Part model, mm, in its own coordinate system. Face numbers are marked on the shaded views. A direction names the side the tool comes from. Round coordinates to 2 decimals unless told otherwise and drop trailing zeros. Loops run counter-clockwise (first coordinate to the right, second up) from the corner with the lowest first, then second, coordinate; pieces in that order, holes last. Notation, with made-up numbers: (-34, 4.5) - (3, 4.5) arc R12 ccw to (3, 8.5) - close; hole circle Ø9 at (19.5, 64). An arc over 180 degrees is marked (long way). Put each result on its own line as item: value.
from build123d import *

# Parameters (mm, degrees)
CUT_EXTRUDE1_DEPTH = 15


with BuildPart() as part:
    # Sketch1 → Revolve1 (revolve)
    with BuildSketch(Plane.XY):
        Polygon((-3, 0), (-3, 7), (-9, 7), (0, 40), (0, 0), align=None)
    revolve(axis=Axis((0, 40, 0), (0, -1, 0)))

    # Sketch2 → Cut-Extrude1 (cut)
    with BuildSketch(Plane.XZ.offset(-7)):
        with BuildLine():
            Line((-2.079651877, 8.756428956), (0, 5.274248167))
            Line((0, 5.274248167), (2.079651877, 8.756428956))
            ThreePointArc((2.079651877, 8.756428956), (0, 9.330174076), (-2.079651877, 8.756428956))
        make_face()
        with BuildLine():
            Line((8.756428956, 2.079651877), (5.274248167, 0))
            Line((5.274248167, 0), (8.756428956, -2.079651877))
            ThreePointArc((8.756428956, -2.079651877), (9.330174076, 0), (8.756428956, 2.079651877))
        make_face()
        with BuildLine():
            Line((2.079651877, -8.756428956), (0, -5.274248167))
            Line((0, -5.274248167), (-2.079651877, -8.756428956))
            ThreePointArc((-2.079651877, -8.756428956), (0, -9.330174076), (2.079651877, -8.756428956))
        make_face()
        with BuildLine():
            Line((-8.756428956, -2.079651877), (-5.274248167, 0))
            Line((-5.274248167, 0), (-8.756428956, 2.079651877))
            ThreePointArc((-8.756428956, 2.079651877), (-9.330174076, 0), (-8.756428956, -2.079651877))
        make_face()
    extrude(amount=-CUT_EXTRUDE1_DEPTH, mode=Mode.SUBTRACT)


solid = part.part
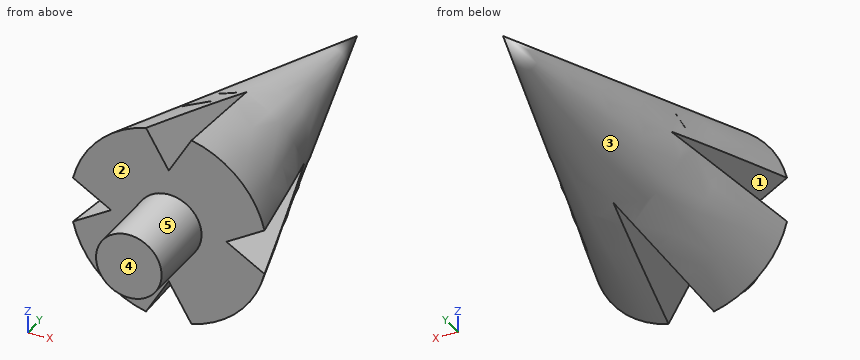
1. Tool access for the marked faces 4 and 5: list every direction of +Z, -Z, +X, -X, +Y, -Y with a clear straight run to the whole face (end or side of a thin tool).
A:
face 4: +Z, -Z, +X, -X, -Y
face 5: -Y
2. Band-saw the part on A-A (y = 9.5). List the corners of the cut face in (x, z).
A:
outline: (-8.14, -1.71) arc R8.32 ccw to (-1.71, -8.14) - (0, -5.27) - (1.71, -8.14) arc R8.32 ccw to (8.14, -1.71) - (5.27, 0) - (8.14, 1.71) arc R8.32 ccw to (1.71, 8.14) - (0, 5.27) - (-1.71, 8.14) arc R8.32 ccw to (-8.14, 1.71) - (-5.27, 0) - close
3. Two-plate mould, pull along Z, no slides. Class the marked faces 1, 2 and 3: pulls with the +Z half, pulls with the -Z half, needs draft (parallel to the pull), parting line crosses it, or undercut.
A:
face 1: undercut
face 2: needs draft
face 3: parting line crosses it
4. Band-saw the part on C-C (y = 28.5). List the corners of the cut face in (x, z), plus the area to 3 significant figures.
A:
outline: circle Ø6.27 at (0, 0)
area: 30.9 mm²
5. Band-saw the part on B-B (y = 14). List the corners of the cut face in (x, z), plus the area to 3 significant figures.
A:
outline: (-7.01, -1.04) arc R7.09 ccw to (-1.04, -7.01) - (0, -5.27) - (1.04, -7.01) arc R7.09 ccw to (7.01, -1.04) - (5.27, 0) - (7.01, 1.04) arc R7.09 ccw to (1.04, 7.01) - (0, 5.27) - (-1.04, 7.01) arc R7.09 ccw to (-7.01, 1.04) - (-5.27, 0) - close
area: 150 mm²
6. Pin check, flat tips, straight feed: P1, Ø8, axis at x = -6.5, y = 15, coming from the +Z side; P2, Ø10, axis at x = 1.5, y = 14.5, coming from the +Z side; P3, Ø1.5, axis at x = -2, y = 24, coming from the +Z side. Stop position of each tip, or through.
A:
P1: stops at z = 6.71
P2: stops at z = 8.14
P3: stops at z = 4.26
7. Probe line 1 along Z through (x, y) = (6.25, 10); line 2 along X through (y, z) = (4.5, 0); line 3 along X through (y, z) = (7.5, -6). List the from-to ranges inside material, lowest first. Write a range as [from, to].
A:
line 1: z = [-5.28, -0.58], [0.58, 5.28]
line 2: x = [-3, 3]
line 3: x = [-6.52, -0.43], [0.43, 6.52]
